Read the model definition and answer for the solid it produces. Units are mm, in the model's axes. A direction names the side the tool comes from. Give positions to 0.01 mm unless a question says otherwise; leave off trailing zeros. Order: outer loops, then holes, each group sorted by start corner. A loop starts at its lowest first (then second) coordinate and runs counter-clockwise, first axis right, second up. Notation, with made-up numbers: M 38.25,-13 L 85.25,-13 A9 ccw 85.25,3 Z; hole C -37,64.5 d8. An arc over 180 degrees is marked long. Write item = value, one per line. Start each with the question number.
Autodesk Inventor part; units mm, degrees
ref_plane "MSC_PF1" through (0, 0, 0) normal (1, 0, 0) x (0, 1, 0)
ref_plane "MSC_PT1" through (0, 0, 0) normal (0, 0, -1) x (-1, 0, 0)
ref_plane "YZ Plane" through (0, 0, 0) normal (1, 0, 0) x (0, 1, 0)
sketch "Sketch1" plane through (0, 0, 0) normal (0, 1, 0) x (-1, 0, 0)
  point P0 (0, 0)
sketch "Sketch2" plane through (0, 0, 0) normal (0, 1, 0) x (-1, 0, 0)
  line L0 (-2.5, -20) -> (0, -20)
  line L1 (-2.5, -2.8) -> (-2.5, -20)
  line L2 (-5, -0.3) -> (-2.5, -2.8)
  line L3 (-5, 0) -> (-5, -0.3)
  line L4 (0, 0) -> (-5, 0)
  line L5 (0, -20) -> (0, 0)
  line L6 (0, -20) -> (0, 0)
  line L7 (0, -24) -> (0, 4)
  line L8 (1, 0) -> (-6, 0)
  dimension "d3" = 5
  dimension "d5" = 2.5
  dimension "d7" = 20
  dimension "ParC" = 0.3
  dimension "d22" = 0
  dimension "d23" = 0
  dimension "d43" = 45
revolve "Revolution1" add sketch "Sketch2" angle 360 about axis through (0, 0, -20) along (0, 0, -1)
sketch "Sketch3" plane through (0, 0, 0) normal (0, 0, 1) x (1, 0, 0)
  line L0 (-1.5, 0.866) -> (-1.5, -0.866)
  line L1 (0, 1.7321) -> (-1.5, 0.866)
  line L2 (1.5, 0.866) -> (0, 1.7321)
  line L3 (1.5, -0.866) -> (1.5, 0.866)
  line L4 (0, -1.7321) -> (1.5, -0.866)
  line L5 (-1.5, -0.866) -> (0, -1.7321)
  circle A0 centre (0, 0) radius 1.5 construction
  circle A1 centre (0, 0) radius 2.5 construction
  dimension "d11" = 3
  dimension "d13" = 120
  dimension "d15" = 120
extrude "Extrusion1" cut sketch "Sketch3" against normal blind 2.3
fillet "Fillet1" radius 0.2 1 edges at (-2.5, 0, -2.8)
chamfer "Chamfer1" distance 0.4 angle 45 1 edges at (-2.5, 0, -20) measured on face at (-0.599, -2.4272, -14.2943)
thread "Thread1"
ref_plane "MSC_PF1" through (0, 0, 0) normal (1, 0, 0) x (0, 1, 0)
ref_plane "MSC_PT1" through (0, 0, 0) normal (0, 0, -1) x (-1, 0, 0)
equation "\"d3\" = 0.5 * dk"
equation "\"d5\" = 0.5 * NND"
equation "\"d7\" = NLG"
equation "\"d43\" = 0.5 * ang"
equation "\"d18\" = r"
equation "\"d19\" = 0.5 * PTC"
equation "\"d39\" = 0.5 * PTC"
equation "\"d11\" = ParS"
equation "\"d16\" = ParT"
equation "\"NND\" = 5"
equation "\"PTC\" = 0.8"
equation "\"ParK\" = 2.8"
equation "\"ParS\" = 3"
equation "\"ParT\" = 2.3"
equation "\"r\" = 0.2"
equation "\"NLG\" = 20"
equation "\"ang\" = 90deg"
equation "\"THREADDIA\" = NND"
properties part number "DIN 7991 - M5x20" material "Steel, Mild"
1) Find the intervals of material crossed by probe 1 along X at (y, z) = (-2, -10.75); probe 2 along Z at (x, y) = (-0.75, -0.75); probe 3 along Y at (x, z) = (-1.25, -1.75), in increasing order. Write a range as [from, to].
2) For faces 4 (the face through (0, 0, -20)), 5 (the face through (-0.54, 2.44, -11.36)), 6 (the face through (0.74, -1.305, -1.134)), determine the directions among +Z, -Z, +X, -X, +Y, -Y from which every point of the face is accessible in a straight line to the end or side of a thin tool.
3) For a pull along X with two mould halves and no side action, classify faces 1 (the face through (2.586, 0.814, -2.589)), 2 (the face through (2, 0, 0)), 3 (the face through (-0.74, 1.305, -1.134)) as pulls with the +X half, pulls with the -X half, needs draft (parallel to the pull), parting line crosses it, or undercut.
4) Find section A-A on z = -4. Determine the outline of the cut face in (x, y).
5) Each of these flat-tipped pins is pushed along its axis until it touches: P1, Ø3, axis at x = -2, z = -8.5, coming from the -Y side; P2, Ø3, axis at x = 3, z = -7.5, coming from the +Y side; P3, Ø5, axis at y = -0.5, z = -4, coming from the +X side. Where does it stop, or does it pass through?
Numbers:
q1.probe_1 = [-1.5, 1.5]
q1.probe_2 = [-20, -2.3]
q1.probe_3 = [-3.32, -1.01], [1.01, 3.32]
q2.face_4 = -Z, +X, -X, +Y, -Y
q2.face_5 = -Z
q2.face_6 = +Z
q3.face_1 = parting line crosses it
q3.face_2 = needs draft
q3.face_3 = undercut
q4.outline = C 0,0 d5
q5.P1 = -2.45
q5.P2 = 2
q5.P3 = 3.78
